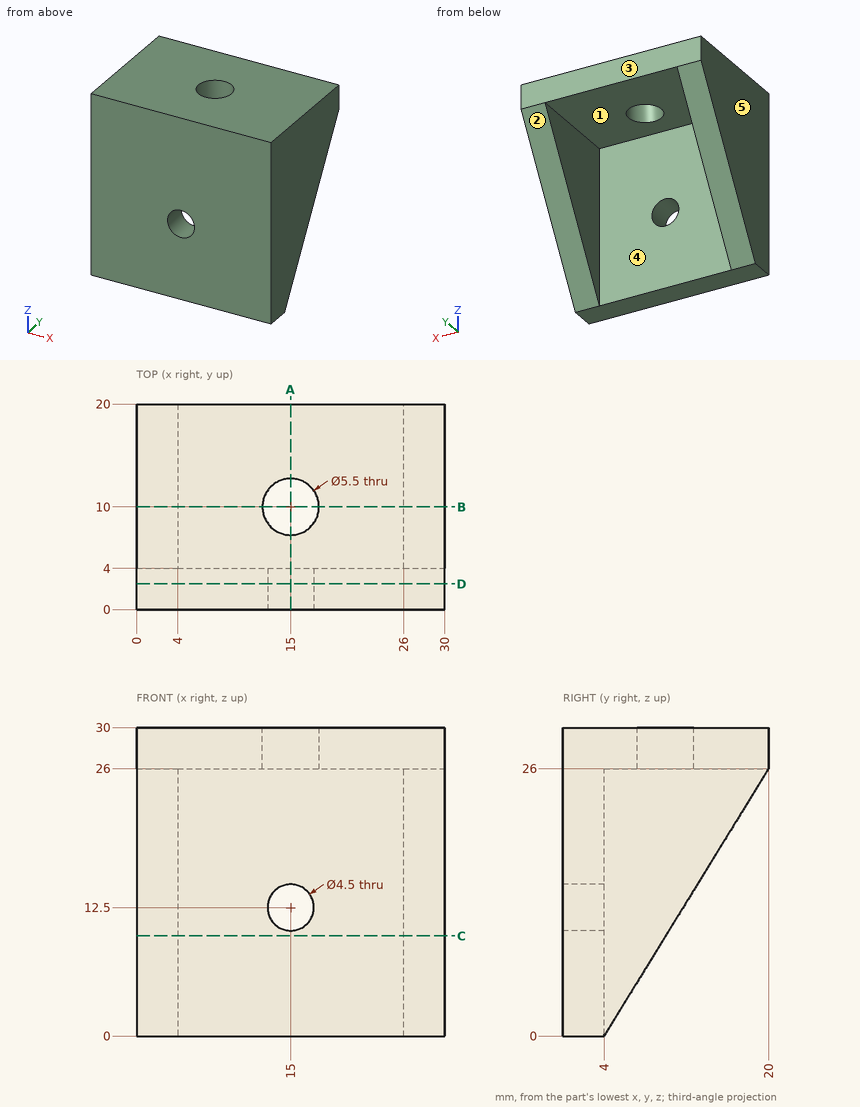
The figure shows three views and two pictorial views of one solid part (mm, origin at its lowest corner). Answer the questions. A direction names the side the tool comes from. Coordinates: 2 decimals unless noted, no trailing zeros. Loops run counter-clockwise (first coordinate to the right, second up) from the corner with the lowest first, then second, coordinate; pieces in that order, holes last. Notation, with made-up numbers: (40.5, 49.25) - (84.5, 49.25) arc R19 cw to (84.5, 59.25) - close; hole circle Ø10 at (18.5, -1.5). An arc over 180 degrees is marked (long way). Use a Markdown table: item, result. Add a question column.
1) Find the intervals of material crossed by line 1 (X direction, y = 12.75, z = 21.25); line 2 (Y direction, x = 15, z = 28); line 3 (X direction, y = 3.15, z = 12.5), in increasing order.
2) The part is cut by section B-B, the plane y = 10. Give the vertices of the cut face in (x, z).
3) Given pin 1 (3 mm diameter, centred on x = 14.5, z = 21.5, fed in from +Y); pin 2 (6 mm diameter, centred on x = 15, z = 12.5, fed in from -Y); pin 3 (8 mm diameter, centred on x = 11, y = 14.5, fed in from -Z); pin 4 (3 mm diameter, centred on x = 26.5, y = 13, fed in from -Z), each flat-ended and moving along its own axis, determine where each tip first touches the part or whether it passes through.
4) The part is cut by section C-C, the plane z = 9.75. Give the vertices of the cut face in (x, y).
5) The part is cut by section D-D, the plane y = 2.5. Give the vertices of the cut face in (x, z).
6) For the marked faces 1 and 2, determine the directions among +Z, -Z, +X, -X, +Y, -Y from which every point of the face is accessible in a straight line to the end or side of a thin tool.
7) The part is cut by section A-A, the plane x = 15. Give the vertices of the cut face in (y, z).
8) The mould has two halves that part along X. Classify the marked faces 3, 4 and 5: released by +X, released by -X, zero draft, split by the parting line, or undercut.
Here are the results:
| question | item | result |
|---|---|---|
| 1 | line 1 | x = 0 to 4, 26 to 30 |
| 1 | line 2 | y = 0 to 7.25, 12.75 to 20 |
| 1 | line 3 | x = 0 to 12.75, 17.25 to 30 |
| 2 | outline | (0, 9.75) - (4, 9.75) - (4, 26) - (12.25, 26) - (12.25, 30) - (0, 30) - close; (17.75, 26) - (26, 26) - (26, 9.75) - (30, 9.75) - (30, 30) - (17.75, 30) - close |
| 3 | pin 1 | stops at y = 4 |
| 3 | pin 2 | stops at y = 0 |
| 3 | pin 3 | stops at z = 26 |
| 3 | pin 4 | stops at z = 12.19 |
| 4 | outline | (0, 0) - (30, 0) - (30, 10) - (26, 10) - (26, 4) - (4, 4) - (4, 10) - (0, 10) - close |
| 5 | outline | (0, 0) - (30, 0) - (30, 30) - (0, 30) - close; hole circle Ø4.5 at (15, 12.5) |
| 6 | face 1 | -Z, +Y |
| 6 | face 2 | -Z, +X, -X, +Y |
| 7 | outline | (0, 0) - (4, 0) - (4, 10.25) - (0, 10.25) - close; (0, 14.75) - (4, 14.75) - (4, 26) - (7.25, 26) - (7.25, 30) - (0, 30) - close; (12.75, 26) - (20, 26) - (20, 30) - (12.75, 30) - close |
| 8 | face 3 | zero draft |
| 8 | face 4 | undercut |
| 8 | face 5 | released by -X |
